```python
from build123d import *

# Parameters (mm, degrees)
SKETCH2_W           = 9.5
SKETCH2_H           = 11.35
BOSS_EXTRUDE1_DEPTH = 12
SKETCH3_R           = 3.5
BOSS_EXTRUDE2_DEPTH = 5
SKETCH4_R           = 3
BOSS_EXTRUDE3_DEPTH = 10
SKETCH5_W           = 10
SKETCH5_H           = 1
CUT_EXTRUDE1_DEPTH  = 9
SKETCH6_W           = 2
SKETCH6_H           = 0.7
BOSS_EXTRUDE4_DEPTH = 0.8
SKETCH7_R           = 0.5
BOSS_EXTRUDE5_DEPTH = 3.5


with BuildPart() as part:
    # Sketch2 → Boss-Extrude1 (new body)
    with BuildSketch(Plane(origin=(0, 0, 0), x_dir=(1, 0, 0), z_dir=(0, 1, 0))):
        with Locations((0, -0.825)):
            Rectangle(SKETCH2_W, SKETCH2_H)
    extrude(amount=-BOSS_EXTRUDE1_DEPTH)

    # Sketch3 → Boss-Extrude2 (add)
    with BuildSketch(Plane(origin=(0, 0, 0), x_dir=(1, 0, 0), z_dir=(0, 1, 0))):
        with Locations(Location((0, 0, 0), (0, 0, 270))):
            Circle(SKETCH3_R)
    extrude(amount=BOSS_EXTRUDE2_DEPTH)

    # Sketch4 → Boss-Extrude3 (add)
    with BuildSketch(Plane(origin=(0, 5, 0), x_dir=(1, 0, 0), z_dir=(0, 1, 0))):
        with Locations(Location((0, 0, 0), (0, 0, 270))):
            Circle(SKETCH4_R)
    extrude(amount=BOSS_EXTRUDE3_DEPTH)

    # Sketch5 → Cut-Extrude1 (cut)
    with BuildSketch(Plane(origin=(0, 15, 0), x_dir=(1, 0, 0), z_dir=(0, 1, 0))):
        Rectangle(SKETCH5_W, SKETCH5_H)
    extrude(amount=-CUT_EXTRUDE1_DEPTH, mode=Mode.SUBTRACT)

    # Sketch6 → Boss-Extrude4 (add)
    with BuildSketch(Plane(origin=(0, 0, 0), x_dir=(1, 0, 0), z_dir=(0, 1, 0))):
        with Locations((0, -6.15)):
            Rectangle(SKETCH6_W, SKETCH6_H)
    extrude(amount=BOSS_EXTRUDE4_DEPTH)

    # Sketch7 → Boss-Extrude5 (add)
    with BuildSketch(Plane.XY.offset(6.5)):
        with Locations((-2.5, -4.3)):
            Circle(SKETCH7_R)
        with Locations((0, -4.3)):
            Circle(SKETCH7_R)
        with Locations((2.5, -4.3)):
            Circle(SKETCH7_R)
        with Locations((0, -10.6)):
            Circle(SKETCH7_R)
        with Locations((2.5, -10.6)):
            Circle(SKETCH7_R)
        with Locations((-2.5, -10.6)):
            Circle(SKETCH7_R)
    extrude(amount=BOSS_EXTRUDE5_DEPTH)


solid = part.part
```
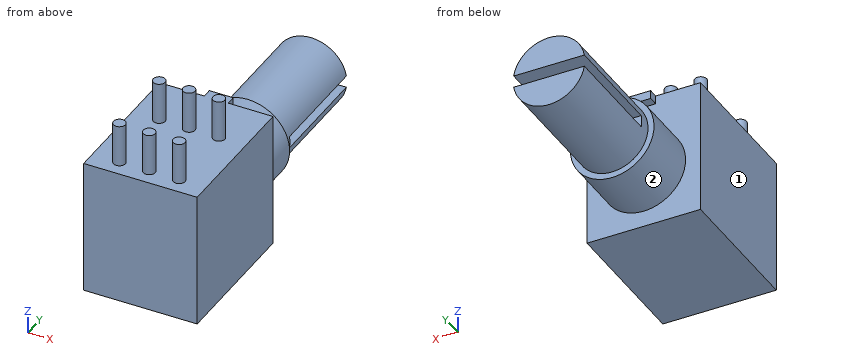
Here's how the part is built. I have some questions about the finished solid (model axes, mm). Face numbers are marked on the shaded views. A direction names the side the tool comes from. Give positions to 0.01 mm unless a question says otherwise; leave off trailing zeros. Write each loop counter-clockwise with the first axis right and the second up, starting at its lowest first coordinate (ties: lowest second). Pieces come first, ordered by that corner, then holes. Notation, with made-up numbers: M 39.25,74 L 98.25,74 A30 ccw 98.25,112 Z; hole C 42,40.5 d2. An arc over 180 degrees is marked long. Put each result on its own line as item: value. Start each with the question number.
Item 1: Will these pins go through, and if not, where does the flat tip stop? pin 1 (0.8 mm diameter, centred on x = 0, z = 0, fed in from +Y); pin 2 (4.5 mm diameter, centred on x = -0.5, y = 10, fed in from -Z); pin 3 (5 mm diameter, centred on x = -1, y = 8, fed in from +Z); pin 4 (4 mm diameter, centred on y = 6, z = 6, fed in from +X).
Item 2: On a 3-axis mill with a long thin cutter (end or side, diameter ignored), from which of +Z, -Z, +X, -X, +Y, -Y can I reach the whole of each face in a straight line? I mean the marked faces 1 and 2. Say none if no direction works.
Item 3: If we section it at A-A, the plane x = 0: Write out the boundary of the cut face in (y, z).
Item 4: I need wall thicknesses on L1, parallel to Z at x = 0.5, y = -3; L2, parallel to Y at x = 0.75, z = 4; L3, parallel to Y at x = -1.25, z = -0.25. Which ranges of each line are inside material? Lowest first, please. Write a range as from..to.
Item 5: If we section it at B-B, the plane y = -10.6: Write out the boundary of the cut face in (x, z).
Item 6: If we section it at C-C, the plane z = 0: Write out the boundary of the cut face in (x, y).
Item 7: If we section it at D-D, the plane y = 8.5: Write out the boundary of the cut face in (x, z), then the cut area to 3 significant figures.
Values:
1. pin 1: y = 6
1. pin 2: z = -3
1. pin 3: z = 3
1. pin 4: through
2. face 1: +Z, -Z, -X, +Y, -Y
2. face 2: +Y
3. outline: M -12,-4.85 L 0,-4.85 L 0,-3.5 L 5,-3.5 L 5,-3 L 15,-3 L 15,-0.5 L 6,-0.5 L 6,0.5 L 15,0.5 L 15,3 L 5,3 L 5,3.5 L 0,3.5 L 0,5.8 L 0.8,5.8 L 0.8,6.5 L -3.8,6.5 L -3.8,10 L -4.8,10 L -4.8,6.5 L -10.1,6.5 L -10.1,10 L -11.1,10 L -11.1,6.5 L -12,6.5 Z
4. L1: -4.85..6.5
4. L2: -12..0
4. L3: -12..6
5. outline: M -4.75,-4.85 L 4.75,-4.85 L 4.75,6.5 L 3,6.5 L 3,10 L 2,10 L 2,6.5 L 0.5,6.5 L 0.5,10 L -0.5,10 L -0.5,6.5 L -2,6.5 L -2,10 L -3,10 L -3,6.5 L -4.75,6.5 Z
6. outline: M -4.75,-12 L 4.75,-12 L 4.75,0 L 3.5,0 L 3.5,5 L 3,5 L 3,6 L -3,6 L -3,5 L -3.5,5 L -3.5,0 L -4.75,0 Z
7. outline: M -2.96,-0.5 A3 ccw 2.96,-0.5 Z; M -2.96,0.5 L 2.96,0.5 A3 ccw Z
7. area: 22.3 mm²
